Work out the finished part from the listing and answer in its coordinate system (mm). Coordinates: 2 decimals unless noted, no trailing zeros. Order: outer loops, then holes, each group sorted by start corner. A loop starts at its lowest first (then second) coordinate and runs counter-clockwise, first axis right, second up. Notation, with made-up numbers: M 63,-27 L 122,-27 A18 ccw 122,7 Z; hole C 47.5,31.25 d8. An arc over 180 degrees is marked long. Use a Markdown table: item, result.
from build123d import *

# Parameters (mm, degrees)
SKETCH1_W             = 82
SKETCH1_H             = 124
SKETCH1_W_2           = 44
SKETCH1_H_2           = 54
SKETCH1_W_3           = 10
SKETCH1_H_3           = 102
SKETCH1_W_4           = 14
SKETCH1_H_4           = 74
SKETCH1_W_5           = 30
SKETCH1_H_5           = 15
BOSS_EXTRUDE1_DEPTH   = 10
FILLET1_R             = 3
FILLET2_R             = 2
FILLET3_R             = 5
FILLET4_R             = 2
FILLET5_R             = 3
CHAMFER1_SIZE         = 5
FILLET6_R             = 5
SKETCH2_W             = 58
SKETCH2_H             = 165
CUT_EXTRUDE1_DEPTH    = 5.5
SKETCH3_W             = 58
SKETCH3_H             = 100
CUT_EXTRUDE2_DEPTH    = 5.5
FILLET7_R             = 3
FILLET8_R             = 5
SKETCH4_R             = 2
CUT_EXTRUDE3_DEPTH    = 11
M4_TAPPED_HOLE1_D     = 3.3
M4_TAPPED_HOLE1_DEPTH = 8
M4_TAPPED_HOLE1_TIP   = 0.991420021
M4_TAPPED_HOLE2_D     = 3.3
M4_TAPPED_HOLE2_DEPTH = 8
M4_TAPPED_HOLE2_TIP   = 0.991420021
M10_TAPPED_HOLE1_D    = 8.5
M4_TAPPED_HOLE3_D     = 3.3
M4_TAPPED_HOLE3_DEPTH = 10.1
M4_TAPPED_HOLE3_TIP   = 0.991420021
SKETCH15_R            = 2
CUT_EXTRUDE4_DEPTH    = 11
M3_TAPPED_HOLE1_D     = 2.5
M3_TAPPED_HOLE1_DEPTH = 7.5
M3_TAPPED_HOLE1_TIP   = 0.751075774
M6_TAPPED_HOLE1_D     = 5
M6_TAPPED_HOLE1_DEPTH = 15
M6_TAPPED_HOLE1_TIP   = 1.502151548


with BuildPart() as part:
    # Sketch1 → Boss-Extrude1 (new body)
    with BuildSketch(Plane.XY):
        Polygon((-81.731872987, 190.622065728), (543.268127013, 190.622065728), (543.268127013, -341.377934272), (168.268127013, -341.377934272), (168.268127013, -139.377934272), (-81.731872987, -139.377934272), align=None)
        with Locations((21.268127013, 108.622065728)):
            Rectangle(SKETCH1_W, SKETCH1_H, mode=Mode.SUBTRACT)
        with Locations((394.268127013, -209.877934272)):
            Rectangle(SKETCH1_W_2, SKETCH1_H_2, mode=Mode.SUBTRACT)
        with Locations((-12.731872987, -30.377934272)):
            Rectangle(SKETCH1_W_3, SKETCH1_H_3, mode=Mode.SUBTRACT)
        with BuildLine():
            Line((110.768127013, 102.622065728), (110.768127013, 90.622065728))
            ThreePointArc((110.768127013, 90.622065728), (118.268127013, 83.122065728), (125.768127013, 90.622065728))
            Line((125.768127013, 90.622065728), (125.768127013, 102.622065728))
            ThreePointArc((125.768127013, 102.622065728), (118.268127013, 110.122065728), (110.768127013, 102.622065728))
        make_face(mode=Mode.SUBTRACT)
        with BuildLine():
            Line((146.768127013, 102.622065728), (146.768127013, 90.622065728))
            ThreePointArc((146.768127013, 90.622065728), (154.268127013, 83.122065728), (161.768127013, 90.622065728))
            Line((161.768127013, 90.622065728), (161.768127013, 102.622065728))
            ThreePointArc((161.768127013, 102.622065728), (154.268127013, 110.122065728), (146.768127013, 102.622065728))
        make_face(mode=Mode.SUBTRACT)
        with Locations((360.268127013, -123.377934272)):
            Rectangle(SKETCH1_W_4, SKETCH1_H_4, mode=Mode.SUBTRACT)
        with Locations((422.268127013, -296.377934272)):
            Rectangle(SKETCH1_W_4, SKETCH1_H_4, mode=Mode.SUBTRACT)
        with Locations((403.268127013, 36.122065728)):
            Rectangle(SKETCH1_W_5, SKETCH1_H_5, mode=Mode.SUBTRACT)
        with Locations((421.268127013, -30.377934272)):
            Rectangle(SKETCH1_W_3, SKETCH1_H_3, mode=Mode.SUBTRACT)
    extrude(amount=BOSS_EXTRUDE1_DEPTH)

    # Fillet1
    fillet1_edges = [part.edges().sort_by_distance(p)[0] for p in [
        (-19.731872987, 170.622065728, 5),
        (-19.731872987, 46.622065728, 5),
        (62.268127013, 46.622065728, 5),
        (62.268127013, 170.622065728, 5),
    ]]
    fillet(fillet1_edges, radius=FILLET1_R)

    # Fillet2
    fillet2_edges = [part.edges().sort_by_distance(p)[0] for p in [
        (-17.731872987, 20.622065728, 5),
        (-17.731872987, -81.377934272, 5),
        (-7.731872987, -81.377934272, 5),
        (-7.731872987, 20.622065728, 5),
    ]]
    fillet(fillet2_edges, radius=FILLET2_R)

    # Fillet3
    fillet3_edges = [part.edges().sort_by_distance(p)[0] for p in [
        (388.268127013, 43.622065728, 5),
        (388.268127013, 28.622065728, 5),
        (418.268127013, 28.622065728, 5),
        (418.268127013, 43.622065728, 5),
    ]]
    fillet(fillet3_edges, radius=FILLET3_R)

    # Fillet4
    fillet4_edges = [part.edges().sort_by_distance(p)[0] for p in [
        (416.268127013, 20.622065728, 5),
        (416.268127013, -81.377934272, 5),
        (426.268127013, -81.377934272, 5),
        (426.268127013, 20.622065728, 5),
    ]]
    fillet(fillet4_edges, radius=FILLET4_R)

    # Fillet5
    fillet5_edges = [part.edges().sort_by_distance(p)[0] for p in [
        (372.268127013, -182.877934272, 5),
        (372.268127013, -236.877934272, 5),
        (416.268127013, -236.877934272, 5),
        (416.268127013, -182.877934272, 5),
        (415.268127013, -259.377934272, 5),
        (415.268127013, -333.377934272, 5),
        (429.268127013, -333.377934272, 5),
        (429.268127013, -259.377934272, 5),
        (353.268127013, -86.377934272, 5),
        (353.268127013, -160.377934272, 5),
        (367.268127013, -160.377934272, 5),
        (367.268127013, -86.377934272, 5),
    ]]
    fillet(fillet5_edges, radius=FILLET5_R)

    # Chamfer1
    chamfer1_edges = [part.edges().sort_by_distance(p)[0] for p in [
        (-81.731872987, 190.622065728, 5),
        (543.268127013, 190.622065728, 5),
        (543.268127013, -341.377934272, 5),
        (168.268127013, -341.377934272, 5),
        (-81.731872987, -139.377934272, 5),
    ]]
    chamfer(chamfer1_edges, length=CHAMFER1_SIZE)

    # Fillet6
    fillet6_edges = [part.edges().sort_by_distance(p)[0] for p in [
        (168.268127013, -139.377934272, 5),
    ]]
    fillet(fillet6_edges, radius=FILLET6_R)

    # Sketch2 → Cut-Extrude1 (cut)
    with BuildSketch(Plane.XY.offset(10)):
        with Locations((136.268127013, -11.877934272)):
            Rectangle(SKETCH2_W, SKETCH2_H)
    extrude(amount=-CUT_EXTRUDE1_DEPTH, mode=Mode.SUBTRACT)

    # Sketch3 → Cut-Extrude2 (cut, through all)
    with BuildSketch(Plane.XY.offset(4.5)):
        with Locations((136.268127013, -44.377934272)):
            Rectangle(SKETCH3_W, SKETCH3_H)
    extrude(amount=-CUT_EXTRUDE2_DEPTH, mode=Mode.SUBTRACT)

    # Fillet7
    fillet7_edges = [part.edges().sort_by_distance(p)[0] for p in [
        (107.268127013, -94.377934272, 5),
        (107.268127013, 70.622065728, 7.25),
        (165.268127013, 70.622065728, 7.25),
        (165.268127013, -94.377934272, 5),
    ]]
    fillet(fillet7_edges, radius=FILLET7_R)

    # Fillet8
    fillet8_edges = [part.edges().sort_by_distance(p)[0] for p in [
        (165.268127013, 5.622065728, 2.25),
        (107.268127013, 5.622065728, 2.25),
    ]]
    fillet(fillet8_edges, radius=FILLET8_R)

    # Sketch4 → Cut-Extrude3 (cut, through all)
    with BuildSketch(Plane.XY.offset(10)):
        with Locations((6.768127013, 37.122065728)):
            Circle(SKETCH4_R)
        with Locations((6.768127013, -73.877934272)):
            Circle(SKETCH4_R)
        with Locations((348.768127013, 37.122065728)):
            Circle(SKETCH4_R)
        with Locations((348.768127013, -73.877934272)):
            Circle(SKETCH4_R)
    extrude(amount=-CUT_EXTRUDE3_DEPTH, mode=Mode.SUBTRACT)

    # M4 Tapped Hole1
    with Locations(Plane.ZY.offset(81.731872987)):
        with Locations((5, 47.622065728), (5, -27.377934272)):
            Hole(M4_TAPPED_HOLE1_D / 2, depth=M4_TAPPED_HOLE1_DEPTH)
            with Locations((0, 0, -(M4_TAPPED_HOLE1_DEPTH + M4_TAPPED_HOLE1_TIP / 2))):  # 118° drill point
                Cone(0, M4_TAPPED_HOLE1_D / 2, M4_TAPPED_HOLE1_TIP, mode=Mode.SUBTRACT)

    # M4 Tapped Hole2
    with Locations(Plane(origin=(543.268127013, 0, 0), x_dir=(0, 0, -1), z_dir=(1, 0, 0))):
        with Locations((-5, 47.622065728), (-5, -27.377934272)):
            Hole(M4_TAPPED_HOLE2_D / 2, depth=M4_TAPPED_HOLE2_DEPTH)
            with Locations((0, 0, -(M4_TAPPED_HOLE2_DEPTH + M4_TAPPED_HOLE2_TIP / 2))):  # 118° drill point
                Cone(0, M4_TAPPED_HOLE2_D / 2, M4_TAPPED_HOLE2_TIP, mode=Mode.SUBTRACT)

    # M10 Tapped Hole1 (through all)
    with Locations(Plane.XY.offset(10)):
        with Locations((118.268127013, -109.377934272), (193.268127013, -269.377934272), (503.268127013, -269.377934272), (118.268127013, 120.622065728), (503.268127013, 120.622065728)):
            Hole(M10_TAPPED_HOLE1_D / 2)

    # M4 Tapped Hole3
    with Locations(Plane.XY.offset(10)):
        with Locations((513.268127013, -55.377934272), (528.268127013, -55.377934272)):
            Hole(M4_TAPPED_HOLE3_D / 2, depth=M4_TAPPED_HOLE3_DEPTH)
            with Locations((0, 0, -(M4_TAPPED_HOLE3_DEPTH + M4_TAPPED_HOLE3_TIP / 2))):  # 118° drill point
                Cone(0, M4_TAPPED_HOLE3_D / 2, M4_TAPPED_HOLE3_TIP, mode=Mode.SUBTRACT)

    # Sketch15 → Cut-Extrude4 (cut, through all)
    with BuildSketch(Plane.XY.offset(10)):
        with Locations((49.768127013, 34.222065728)):
            Circle(SKETCH15_R)
        with Locations((49.768127013, -74.777934272)):
            Circle(SKETCH15_R)
        with Locations((440.268127013, 34.222065728)):
            Circle(SKETCH15_R)
        with Locations((440.268127013, -74.777934272)):
            Circle(SKETCH15_R)
        with Locations((59.768127013, 34.222065728)):
            Circle(SKETCH15_R)
        with Locations((59.768127013, -74.777934272)):
            Circle(SKETCH15_R)
        with Locations((450.268127013, 34.222065728)):
            Circle(SKETCH15_R)
        with Locations((450.268127013, -74.777934272)):
            Circle(SKETCH15_R)
    extrude(amount=-CUT_EXTRUDE4_DEPTH, mode=Mode.SUBTRACT)

    # M3 Tapped Hole1
    with Locations(Plane.XY.offset(10)):
        with Locations((204.768127013, -95.377934272), (212.768127013, -95.377934272)):
            Hole(M3_TAPPED_HOLE1_D / 2, depth=M3_TAPPED_HOLE1_DEPTH)
            with Locations((0, 0, -(M3_TAPPED_HOLE1_DEPTH + M3_TAPPED_HOLE1_TIP / 2))):  # 118° drill point
                Cone(0, M3_TAPPED_HOLE1_D / 2, M3_TAPPED_HOLE1_TIP, mode=Mode.SUBTRACT)

    # M6 Tapped Hole1
    with Locations(Plane.XY.offset(10)):
        with Locations((124.268127013, 162.622065728), (156.268127013, 162.622065728), (124.268127013, 132.622065728), (156.268127013, 132.622065728)):
            Hole(M6_TAPPED_HOLE1_D / 2, depth=M6_TAPPED_HOLE1_DEPTH)
            with Locations((0, 0, -(M6_TAPPED_HOLE1_DEPTH + M6_TAPPED_HOLE1_TIP / 2))):  # 118° drill point
                Cone(0, M6_TAPPED_HOLE1_D / 2, M6_TAPPED_HOLE1_TIP, mode=Mode.SUBTRACT)


solid = part.part
(1) Determine the mould class of faces 1 (the flat face through (136, 36, 4.5)), 2 (the flat face through (305, -72, 10)) for opening direction Y: pulls with the +Y half, pulls with the -Y half, needs draft (parallel to the pull), parting line crosses it, or undercut.
Conclusion:
| item | result |
|---|---|
| face 1 | undercut |
| face 2 | needs draft |
(2) Given P1, Ø2, axis at y = 47.62, z = 5, coming from the +X side; P2, Ø4, axis at y = -240.5, z = 7, coming from the -X side, each flat-ended and moving along its own axis, determine where each tip first touches the part or whether it passes through.
Conclusion:
| item | result |
|---|---|
| P1 | x = 534.88 |
| P2 | x = 168.27 |
(3) Straight lines are drawn through the part: L1, parallel to X at y = 54.5, z = 5; L2, parallel to X at y = 98.5, z = 9; L3, parallel to Y at x = 6.5, z = 5.5. For each, find the intervals that lie inside material, in ascending order.
Conclusion:
| item | result |
|---|---|
| L1 | -81.73 to -19.73, 62.27 to 107.27, 165.27 to 543.27 |
| L2 | -81.73 to -19.73, 62.27 to 110.77, 125.77 to 146.77, 161.77 to 543.27 |
| L3 | -139.38 to -75.86, -71.9 to 35.14, 39.1 to 46.62, 170.62 to 190.62 |
(4) A cutting plane is placed at A-A (y = -214.5). Determine the outline of the cut face in (x, z), then the cut area to 3 significant figures.
Conclusion:
| item | result |
|---|---|
| outline | M 168.27,0 L 372.27,0 L 372.27,10 L 168.27,10 Z; M 416.27,0 L 543.27,0 L 543.27,10 L 416.27,10 Z |
| area | 3,310 mm2 |
